CAD build for the part. Positions are in the model's coordinates, mm. Face numbers are marked on the shaded views. A direction names the side the tool comes from. Coordinates: 2 decimals unless noted, no trailing zeros. Order: outer loops, then holes, each group sorted by start corner. A loop starts at its lowest first (then second) coordinate and runs counter-clockwise, first axis right, second up.
from build123d import *

# Parameters (mm, degrees)
PAD_DEPTH       = 70
SKETCH001_R     = 2.6
POCKET_DEPTH    = 16.870811
SKETCH002_R     = 5
POCKET001_DEPTH = 11.870811
SKETCH003_R     = 1.95
POCKET002_DEPTH = 28.12229
SKETCH004_R     = 1.95
POCKET003_DEPTH = 28.12229
POCKET004_DEPTH = 21.37229
POCKET005_DEPTH = 21.37229
CHAMFER_SIZE    = 1


with BuildPart() as part:
    # Sketch → Pad (new body)
    with BuildSketch(Plane.XZ):
        with BuildLine():
            Line((-12.5, 0), (-4, 0))
            Line((-4, 0), (0, 2))
            Line((0, 2), (4, 0))
            Line((4, 0), (12.5, 0))
            Line((12.5, 0), (23.297234, 0))
            Line((27.193332, 14.540439), (23.297234, 0))
            Line((18.5, 16.869811), (27.193332, 14.540439))
            ThreePointArc((-18.5, 16.869811), (0, 11.58092), (18.5, 16.869811))
            Line((-18.5, 16.869811), (-27.193332, 14.540439))
            Line((-27.193332, 14.540439), (-23.297234, 0))
            Line((-12.5, 0), (-23.297234, 0))
        make_face()
    extrude(amount=PAD_DEPTH)

    # Sketch001 (on Face1 of Pad) → Pocket (cut, through all)
    with BuildSketch(Plane(origin=(0, 0, 0), x_dir=(1, 0, 0), z_dir=(0, 0, -1))):
        with Locations((-8, 63.5)):
            Circle(SKETCH001_R)
        with Locations((8, 63.5)):
            Circle(SKETCH001_R)
        with Locations((-8, 31.5)):
            Circle(SKETCH001_R)
        with Locations((8, 31.5)):
            Circle(SKETCH001_R)
    extrude(amount=-POCKET_DEPTH, mode=Mode.SUBTRACT)

    # Sketch002 → Pocket001 (cut, through all)
    with BuildSketch(Plane(origin=(0, 0, 5), x_dir=(1, 0, 0), z_dir=(0, 0, -1))):
        with Locations((-8, 63.5)):
            Circle(SKETCH002_R)
        with Locations((8, 63.5)):
            Circle(SKETCH002_R)
        with Locations((8, 31.5)):
            Circle(SKETCH002_R)
        with Locations((-8, 31.5)):
            Circle(SKETCH002_R)
    extrude(amount=-POCKET001_DEPTH, mode=Mode.SUBTRACT)

    # Sketch003 (on Face15 of Pocket001) → Pocket002 (cut, through all)
    with BuildSketch(Plane(origin=(-5.456718, 0, 20.364748), x_dir=(-0.965926, 0, -0.258819), z_dir=(-0.258819, 0, 0.965926))):
        with Locations((17.5034, 60)):
            Circle(SKETCH003_R)
        with Locations((17.5034, 35)):
            Circle(SKETCH003_R)
        with Locations((17.5034, 10)):
            Circle(SKETCH003_R)
    extrude(amount=-POCKET002_DEPTH, mode=Mode.SUBTRACT)

    # Sketch004 (on Face16 of Pocket002) → Pocket003 (cut, through all)
    with BuildSketch(Plane(origin=(5.456718, 0, 20.364748), x_dir=(-0.965926, 0, 0.258819), z_dir=(0.258819, 0, 0.965926))):
        with Locations((-17.5034, 60)):
            Circle(SKETCH004_R)
        with Locations((-17.5034, 35)):
            Circle(SKETCH004_R)
        with Locations((-17.5034, 10)):
            Circle(SKETCH004_R)
    extrude(amount=-POCKET003_DEPTH, mode=Mode.SUBTRACT)

    # Sketch005 (on DatumPlane) → Pocket004 (cut, through all)
    with BuildSketch(Plane(origin=(3.709689, 0, 13.844748), x_dir=(-0.965926, 0, 0.258819), z_dir=(0.258819, 0, 0.965926))):
        Polygon((-13.5034, 62.309401), (-17.5034, 64.618802), (-21.5034, 62.309401), (-21.5034, 57.690599), (-17.5034, 55.381198), (-13.5034, 57.690599), align=None)
        Polygon((-13.5034, 37.309401), (-17.5034, 39.618802), (-21.5034, 37.309401), (-21.5034, 32.690599), (-17.5034, 30.381198), (-13.5034, 32.690599), align=None)
        Polygon((-13.5034, 12.309401), (-17.5034, 14.618802), (-21.5034, 12.309401), (-21.5034, 7.690599), (-17.5034, 5.381198), (-13.5034, 7.690599), align=None)
    extrude(amount=-POCKET004_DEPTH, mode=Mode.SUBTRACT)

    # Sketch006 (on DatumPlane) → Pocket005 (cut, through all)
    with BuildSketch(Plane(origin=(-3.709689, 0, 13.844748), x_dir=(-0.965926, 0, -0.258819), z_dir=(-0.258819, 0, 0.965926))):
        Polygon((21.5034, 62.309401), (17.5034, 64.618802), (13.5034, 62.309401), (13.5034, 57.690599), (17.5034, 55.381198), (21.5034, 57.690599), align=None)
        Polygon((21.5034, 37.309401), (17.5034, 39.618802), (13.5034, 37.309401), (13.5034, 32.690599), (17.5034, 30.381198), (21.5034, 32.690599), align=None)
        Polygon((21.5034, 12.309401), (17.5034, 14.618802), (13.5034, 12.309401), (13.5034, 7.690599), (17.5034, 5.381198), (21.5034, 7.690599), align=None)
    extrude(amount=-POCKET005_DEPTH, mode=Mode.SUBTRACT)

    # Chamfer
    chamfer_edges = [part.edges().sort_by_distance(p)[0] for p in [
        (-25.245283, -70, 7.27022),
        (-27.193332, -35, 14.540439),
        (-22.846666, -70, 15.705125),
        (-18.5, -35, 16.869811),
        (-22.846666, 0, 15.705125),
        (-25.245283, 0, 7.27022),
        (22.846666, -70, 15.705125),
        (18.5, -35, 16.869811),
        (27.193332, -35, 14.540439),
        (22.846666, 0, 15.705125),
        (25.245283, -70, 7.27022),
        (25.245283, 0, 7.27022),
        (23.297234, -35, 0),
        (0, 0, 11.58092),
        (0, -70, 11.58092),
    ]]
    chamfer(chamfer_edges, length=CHAMFER_SIZE)


solid = part.part
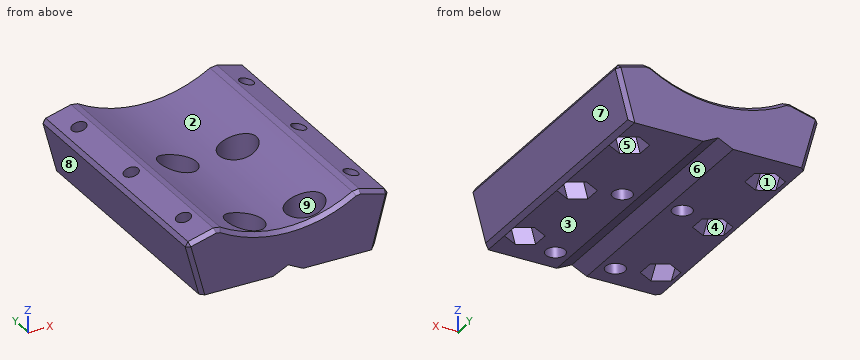
1) Drill centre lines: probe 1 along Y at (x, z) = (-8, 11.5); probe 2 along Y at (x, z) = (-8, 3.7); probe 3 along X at (y, z) = (-63.5, 2.95). Where is each one in solid material? Low to high.
2) Pin check, flat tips, straight feed: P1, Ø11.5, axis at x = 8, y = -63.5, coming from the +Z side; P2, Ø4, axis at x = 16.5, y = -24.5, coming from the +Z side; P3, Ø3, axis at x = 9, y = -61, coming from the +Z side. Stop position of each tip, or through.
3) Slice it at A-A (y = -21). List the corners of the cut face in (x, z).
4) Which spindle directions (+Z, -Z, +X, -X, +Y, -Y) get a long thin tool onto all of the face, cutting with end or side? Do the marked faces 5, 6, 7, 8 and 9. Say none if no direction does.
5) Slice it at B-B (y = -31.5). Give the number of separate pieces and of enclosed holes in the cut face, plus the area to 3 significant figures.
6) Two-plate mould, pull along Z, no slides. Class the marked faces 1, 2, 3 and 4: released by +Z, released by -Z, zero draft, split by the parting line, or undercut.
Worked out:
1. probe 1: y = -69.98 to -68.5, -58.5 to -36.5, -26.5 to -0.02
1. probe 2: y = -70 to -66.1, -60.9 to -34.1, -28.9 to 0
1. probe 3: x = -24.09 to -20.92, -16.91 to -10.6, -5.4 to 5.4, 10.6 to 16.91, 20.92 to 24.09
2. P1: stops at z = 14.39
2. P2: stops at z = 16.47
2. P3: stops at z = 5
3. outline: (-26.93, 13.57) - (-23.3, 0) - (-4, 0) - (0, 2) - (4, 0) - (22.3, 0) - (23.56, 0.97) - (26.93, 13.57) - (26.23, 14.8) - (19.47, 16.61) - (17.64, 16.35) arc R35 cw to (-17.64, 16.35) - (-19.47, 16.61) - (-26.23, 14.8) - close
4. face 5: none
4. face 6: -Z, +Y, -Y
4. face 7: -Z, +X, +Y, -Y
4. face 8: -Z, -X, +Y, -Y
4. face 9: +Z
5. separate pieces: 3
5. enclosed holes: 0
5. area: 418 mm2
6. face 1: undercut
6. face 2: released by +Z
6. face 3: released by -Z
6. face 4: undercut
